Could you check a few things on this model? Use its own coordinates, in mm. A direction names the side the tool comes from. Coordinates: 2 decimals unless noted, no trailing zeros. Loops run counter-clockwise (first coordinate to the right, second up) from the corner with the lowest first, then second, coordinate; pieces in that order, holes last.
from build123d import *

# Parameters (mm, degrees)
SKETCH1_W                    = 80
SKETCH1_H                    = 30
SKETCH1_R                    = 2.5
BASE_FLANGE1_DEPTH           = 2
FILLET1_R                    = 10
EDGE_FLANGE1_STRIP_W         = 14
EDGE_FLANGE1_STRIP_H         = 2
EDGE_FLANGE1_STRIP_CUT_DEPTH = 30
EDGE_FLANGE1_DEPTH           = 30
SKETCH9_W                    = 17
SKETCH9_H                    = 5
CUT_EXTRUDE1_DEPTH           = 10


# Sheet-metal steps are written as plain solids
with BuildPart() as part:
    # Sketch1 → Base-Flange1 (new body)
    with BuildSketch(Plane.XY):
        Rectangle(SKETCH1_W, SKETCH1_H)
        with Locations((30, 0)):
            Circle(SKETCH1_R, mode=Mode.SUBTRACT)
        with Locations((5, 0)):
            Circle(SKETCH1_R, mode=Mode.SUBTRACT)
    extrude(amount=-BASE_FLANGE1_DEPTH)

    # Fillet1
    fillet1_edges = [part.edges().sort_by_distance(p)[0] for p in [
        (40, -15, -1),
        (40, 15, -1),
    ]]
    fillet(fillet1_edges, radius=FILLET1_R)

    # Edge-Flange1 strip (across the edge) → Edge-Flange1 strip cut (cut)
    with BuildSketch(Plane(origin=(-40, 15, 0), x_dir=(1, 0, 0), z_dir=(0, -1, 0))):
        with Locations((-4, -1)):
            Rectangle(EDGE_FLANGE1_STRIP_W, EDGE_FLANGE1_STRIP_H)
    extrude(amount=EDGE_FLANGE1_STRIP_CUT_DEPTH, mode=Mode.SUBTRACT)

    # Edge-Flange1 section (across the edge) → Edge-Flange1 (add)
    with BuildSketch(Plane(origin=(-40, 15, 0), x_dir=(1, 0, 0), z_dir=(0, -1, 0))):
        with BuildLine():
            Line((-2, 3), (-2, 23))
            Line((-2, 23), (0, 23))
            Line((0, 23), (0, 3))
            ThreePointArc((0, 3), (0.878679656, 0.878679656), (3, 0))
            Line((3, 0), (3, -2))
            ThreePointArc((3, -2), (-0.535533906, -0.535533906), (-2, 3))
        make_face()
    extrude(amount=EDGE_FLANGE1_DEPTH)

    # Sketch9 → Cut-Extrude1 (cut)
    with BuildSketch(Plane.ZY.offset(42)):
        with Locations((13.5, 10)):
            Rectangle(SKETCH9_W, SKETCH9_H)
        with Locations((13.5, 0)):
            Rectangle(SKETCH9_W, SKETCH9_H)
        with Locations((13.5, -10)):
            Rectangle(SKETCH9_W, SKETCH9_H)
    extrude(amount=-CUT_EXTRUDE1_DEPTH, mode=Mode.SUBTRACT)


solid = part.part
(1) Imagine slicing it at A-A, the plane z = 8. Write out the boundary of the cut face in (x, y), and give its area (3 significant figures).
Answers:
outline: (-42, -15) - (-40, -15) - (-40, -12.5) - (-42, -12.5) - close; (-42, -7.5) - (-40, -7.5) - (-40, -2.5) - (-42, -2.5) - close; (-42, 2.5) - (-40, 2.5) - (-40, 7.5) - (-42, 7.5) - close; (-42, 12.5) - (-40, 12.5) - (-40, 15) - (-42, 15) - close
area: 30.0 mm2
(2) Imagine slicing it at D-D, the plane y = 9. Write out the boundary of the cut face in (x, z), and give its area (3 significant figures).
Answers:
outline: (-42, 3) arc R5 ccw to (-37, -2) - (39.17, -2) - (39.17, 0) - (-37, 0) arc R3 cw to (-40, 3) - (-40, 5) - (-42, 5) - close; (-42, 22) - (-40, 22) - (-40, 23) - (-42, 23) - close
area: 171 mm2
(3) Which directions (+Z, -Z, +X, -X, +Y, -Y) give clear straight access to the entire face, cutting with the end or side of a thin tool? Please do faces 4 (the face through (1, 0, 0)), 5 (the face through (40, 0, -1)), 6 (the face through (-41, 10, 22)).
Answers:
face 4: +Z, +X, +Y, -Y
face 5: +Z, -Z, +X, +Y, -Y
face 6: +X, -X
(4) Imagine slicing it at B-B, the plane y = 0. Write out the boundary of the cut face in (x, z).
Answers:
outline: (-42, 3) arc R5 ccw to (-37, -2) - (2.5, -2) - (2.5, 0) - (-37, 0) arc R3 cw to (-40, 3) - (-40, 5) - (-42, 5) - close; (-42, 22) - (-40, 22) - (-40, 23) - (-42, 23) - close; (7.5, -2) - (27.5, -2) - (27.5, 0) - (7.5, 0) - close; (32.5, -2) - (40, -2) - (40, 0) - (32.5, 0) - close
(5) Imagine slicing it at C-C, the plane x = 5. Write out the boundary of the cut face in (y, z).
Answers:
outline: (-15, -2) - (-2.5, -2) - (-2.5, 0) - (-15, 0) - close; (2.5, -2) - (15, -2) - (15, 0) - (2.5, 0) - close
(6) I need wall thicknesses on probe 1 along Y at (x, z) = (5, -0.5); probe 2 along Z at (x, y) = (-12, -1); probe 3 along X at (y, z) = (3, 9.5). Which ranges of each line are inside material? Lowest first, please.
Answers:
probe 1: y = -15 to -2.5, 2.5 to 15
probe 2: z = -2 to 0
probe 3: x = -42 to -40
(7) We'd pull the mould along Y, two halves only. Please class faces 1 (the face through (36.99, 12.15, -1.01)), 2 (the face through (-41, 2.5, 13)), 3 (the face through (1, 0, -2)): +Y half, -Y half, draft (parallel to the pull), parting line (faces both ways), or undercut.
Answers:
face 1: +Y half
face 2: undercut
face 3: draft
(8) For pin 1 (2 mm diameter, centred on x = -31, y = 4, fed in from +Z); pin 2 (3 mm diameter, centred on y = -1.5, z = 7, fed in from +X); pin 3 (1 mm diameter, centred on x = -41.5, y = 10.5, fed in from -Z), each with a flat end and sliding along its axis, tell me the tip position at first contact or that it passes through.
Answers:
pin 1: stops at z = 0
pin 2: stops at x = -40
pin 3: stops at z = 0
